```python
from build123d import *

# Parameters (mm, degrees)
SKETCH1_R           = 1
BOSS_EXTRUDE1_DEPTH = 1.5


with BuildPart() as part:
    # Sketch1 → Boss-Extrude1 (new, symmetric)
    with BuildSketch(Plane.XY):
        with BuildLine():
            Line((-0.022308457, 3.388443306), (-0.022308457, 3.09991973))
            ThreePointArc((-0.022308457, 3.09991973), (-0.270182803, 3.088203564), (-0.516325871, 3.056698807))
            Line((-0.516325871, 3.056698807), (-0.566427464, 3.340839061))
            ThreePointArc((-0.566427464, 3.340839061), (-0.583212597, 3.395348635), (-0.607768622, 3.446827136))
            ThreePointArc((-0.607768622, 3.446827136), (-0.806569619, 3.722605346), (-1.04548536, 3.964462178))
            ThreePointArc((-1.04548536, 3.964462178), (-1.402282588, 3.852739745), (-1.747418917, 3.708979257))
            ThreePointArc((-1.747418917, 3.708979257), (-1.774976418, 3.370134097), (-1.75, 3.031088913))
            ThreePointArc((-1.75, 3.031088913), (-1.735721264, 2.975869786), (-1.713541343, 2.923323754))
            Line((-1.713541343, 2.923323754), (-1.569279555, 2.673455008))
            ThreePointArc((-1.569279555, 2.673455008), (-1.778086953, 2.539371337), (-1.975500724, 2.389015883))
            Line((-1.975500724, 2.389015883), (-2.160960104, 2.610037765))
            ThreePointArc((-2.160960104, 2.610037765), (-2.202751242, 2.648851875), (-2.249756634, 2.681155551))
            ThreePointArc((-2.249756634, 2.681155551), (-2.559812453, 2.820585989), (-2.88764797, 2.910582279))
            ThreePointArc((-2.88764797, 2.910582279), (-3.140782217, 2.6354292), (-3.367798802, 2.3383608))
            ThreePointArc((-3.367798802, 2.3383608), (-3.222241717, 2.031133533), (-3.031088913, 1.75))
            ThreePointArc((-3.031088913, 1.75), (-2.991113602, 1.7093182), (-2.945632211, 1.674901963))
            Line((-2.945632211, 1.674901963), (-2.695763464, 1.530640175))
            ThreePointArc((-2.695763464, 1.530640175), (-2.80955414, 1.310116611), (-2.905341754, 1.081198083))
            Line((-2.905341754, 1.081198083), (-3.176465229, 1.179878957))
            ThreePointArc((-3.176465229, 1.179878957), (-3.232064471, 1.192597393), (-3.288924173, 1.197070502))
            ThreePointArc((-3.288924173, 1.197070502), (-3.627155608, 1.162792893), (-3.956067639, 1.076814208))
            ThreePointArc((-3.956067639, 1.076814208), (-4.037711787, 0.711957528), (-4.085779717, 0.341180455))
            ThreePointArc((-4.085779717, 0.341180455), (-3.806109951, 0.14789238), (-3.5, 0))
            ThreePointArc((-3.5, 0), (-3.445039465, -0.015243816), (-3.388443306, -0.022308457))
            Line((-3.388443306, -0.022308457), (-3.09991973, -0.022308457))
            ThreePointArc((-3.09991973, -0.022308457), (-3.088203564, -0.270182803), (-3.056698807, -0.516325871))
            Line((-3.056698807, -0.516325871), (-3.340839061, -0.566427464))
            ThreePointArc((-3.340839061, -0.566427464), (-3.395348635, -0.583212597), (-3.446827136, -0.607768622))
            ThreePointArc((-3.446827136, -0.607768622), (-3.722605346, -0.806569619), (-3.964462178, -1.04548536))
            ThreePointArc((-3.964462178, -1.04548536), (-3.852739745, -1.402282588), (-3.708979257, -1.747418917))
            ThreePointArc((-3.708979257, -1.747418917), (-3.370134097, -1.774976418), (-3.031088913, -1.75))
            ThreePointArc((-3.031088913, -1.75), (-2.975869786, -1.735721264), (-2.923323754, -1.713541343))
            Line((-2.923323754, -1.713541343), (-2.673455008, -1.569279555))
            ThreePointArc((-2.673455008, -1.569279555), (-2.539371337, -1.778086953), (-2.389015883, -1.975500724))
            Line((-2.389015883, -1.975500724), (-2.610037765, -2.160960104))
            ThreePointArc((-2.610037765, -2.160960104), (-2.648851875, -2.202751242), (-2.681155551, -2.249756634))
            ThreePointArc((-2.681155551, -2.249756634), (-2.820585989, -2.559812453), (-2.910582279, -2.88764797))
            ThreePointArc((-2.910582279, -2.88764797), (-2.6354292, -3.140782217), (-2.3383608, -3.367798802))
            ThreePointArc((-2.3383608, -3.367798802), (-2.031133533, -3.222241717), (-1.75, -3.031088913))
            ThreePointArc((-1.75, -3.031088913), (-1.7093182, -2.991113602), (-1.674901963, -2.945632211))
            Line((-1.674901963, -2.945632211), (-1.530640175, -2.695763464))
            ThreePointArc((-1.530640175, -2.695763464), (-1.310116611, -2.80955414), (-1.081198083, -2.905341754))
            Line((-1.081198083, -2.905341754), (-1.179878957, -3.176465229))
            ThreePointArc((-1.179878957, -3.176465229), (-1.192597393, -3.232064471), (-1.197070502, -3.288924173))
            ThreePointArc((-1.197070502, -3.288924173), (-1.162792893, -3.627155608), (-1.076814208, -3.956067639))
            ThreePointArc((-1.076814208, -3.956067639), (-0.711957528, -4.037711787), (-0.341180455, -4.085779717))
            ThreePointArc((-0.341180455, -4.085779717), (-0.14789238, -3.806109951), (0, -3.5))
            ThreePointArc((0, -3.5), (0.015243816, -3.445039465), (0.022308457, -3.388443306))
            Line((0.022308457, -3.388443306), (0.022308457, -3.09991973))
            ThreePointArc((0.022308457, -3.09991973), (0.270182803, -3.088203564), (0.516325871, -3.056698807))
            Line((0.516325871, -3.056698807), (0.566427464, -3.340839061))
            ThreePointArc((0.566427464, -3.340839061), (0.583212597, -3.395348635), (0.607768622, -3.446827136))
            ThreePointArc((0.607768622, -3.446827136), (0.806569619, -3.722605346), (1.04548536, -3.964462178))
            ThreePointArc((1.04548536, -3.964462178), (1.402282588, -3.852739745), (1.747418917, -3.708979257))
            ThreePointArc((1.747418917, -3.708979257), (1.774976418, -3.370134097), (1.75, -3.031088913))
            ThreePointArc((1.75, -3.031088913), (1.735721264, -2.975869786), (1.713541343, -2.923323754))
            Line((1.713541343, -2.923323754), (1.569279555, -2.673455008))
            ThreePointArc((1.569279555, -2.673455008), (1.778086953, -2.539371337), (1.975500724, -2.389015883))
            Line((1.975500724, -2.389015883), (2.160960104, -2.610037765))
            ThreePointArc((2.160960104, -2.610037765), (2.202751242, -2.648851875), (2.249756634, -2.681155551))
            ThreePointArc((2.249756634, -2.681155551), (2.559812453, -2.820585989), (2.88764797, -2.910582279))
            ThreePointArc((2.88764797, -2.910582279), (3.140782217, -2.6354292), (3.367798802, -2.3383608))
            ThreePointArc((3.367798802, -2.3383608), (3.222241717, -2.031133533), (3.031088913, -1.75))
            ThreePointArc((3.031088913, -1.75), (2.991113602, -1.7093182), (2.945632211, -1.674901963))
            Line((2.945632211, -1.674901963), (2.695763464, -1.530640175))
            ThreePointArc((2.695763464, -1.530640175), (2.80955414, -1.310116611), (2.905341754, -1.081198083))
            Line((2.905341754, -1.081198083), (3.176465229, -1.179878957))
            ThreePointArc((3.176465229, -1.179878957), (3.232064471, -1.192597393), (3.288924173, -1.197070502))
            ThreePointArc((3.288924173, -1.197070502), (3.627155608, -1.162792893), (3.956067639, -1.076814208))
            ThreePointArc((3.956067639, -1.076814208), (4.037711787, -0.711957528), (4.085779717, -0.341180455))
            ThreePointArc((4.085779717, -0.341180455), (3.806109951, -0.14789238), (3.5, 0))
            ThreePointArc((3.5, 0), (3.445039465, 0.015243816), (3.388443306, 0.022308457))
            Line((3.388443306, 0.022308457), (3.09991973, 0.022308457))
            ThreePointArc((3.09991973, 0.022308457), (3.088203564, 0.270182803), (3.056698807, 0.516325871))
            Line((3.056698807, 0.516325871), (3.340839061, 0.566427464))
            ThreePointArc((3.340839061, 0.566427464), (3.395348635, 0.583212597), (3.446827136, 0.607768622))
            ThreePointArc((3.446827136, 0.607768622), (3.722605346, 0.806569619), (3.964462178, 1.04548536))
            ThreePointArc((3.964462178, 1.04548536), (3.852739745, 1.402282588), (3.708979257, 1.747418917))
            ThreePointArc((3.708979257, 1.747418917), (3.370134097, 1.774976418), (3.031088913, 1.75))
            ThreePointArc((3.031088913, 1.75), (2.975869786, 1.735721264), (2.923323754, 1.713541343))
            Line((2.923323754, 1.713541343), (2.673455008, 1.569279555))
            ThreePointArc((2.673455008, 1.569279555), (2.539371337, 1.778086953), (2.389015883, 1.975500724))
            Line((2.389015883, 1.975500724), (2.610037765, 2.160960104))
            ThreePointArc((2.610037765, 2.160960104), (2.648851875, 2.202751242), (2.681155551, 2.249756634))
            ThreePointArc((2.681155551, 2.249756634), (2.820585989, 2.559812453), (2.910582279, 2.88764797))
            ThreePointArc((2.910582279, 2.88764797), (2.6354292, 3.140782217), (2.3383608, 3.367798802))
            ThreePointArc((2.3383608, 3.367798802), (2.031133533, 3.222241717), (1.75, 3.031088913))
            ThreePointArc((1.75, 3.031088913), (1.7093182, 2.991113602), (1.674901963, 2.945632211))
            Line((1.674901963, 2.945632211), (1.530640175, 2.695763464))
            ThreePointArc((1.530640175, 2.695763464), (1.310116611, 2.80955414), (1.081198083, 2.905341754))
            Line((1.081198083, 2.905341754), (1.179878957, 3.176465229))
            ThreePointArc((1.179878957, 3.176465229), (1.192597393, 3.232064471), (1.197070502, 3.288924173))
            ThreePointArc((1.197070502, 3.288924173), (1.162792893, 3.627155608), (1.076814208, 3.956067639))
            ThreePointArc((1.076814208, 3.956067639), (0.711957528, 4.037711787), (0.341180455, 4.085779717))
            ThreePointArc((0.341180455, 4.085779717), (0.14789238, 3.806109951), (0, 3.5))
            ThreePointArc((0, 3.5), (-0.015243816, 3.445039465), (-0.022308457, 3.388443306))
        make_face()
        Circle(SKETCH1_R, mode=Mode.SUBTRACT)
    extrude(amount=BOSS_EXTRUDE1_DEPTH, both=True)


solid = part.part
```
Read the model definition and answer for the solid it produces. Units are mm, in the model's axes. Round coordinates to 2 decimals unless told otherwise and drop trailing zeros. Write each loop counter-clockwise with the first axis right and the second up, starting at its lowest first coordinate (ties: lowest second). Pieces come first, ordered by that corner, then holes. Notation, with made-up numbers: (28, 49.5) - (50, 49.5) arc R16 cw to (50, 56.5) - close; hole circle Ø9 at (67, -7). An arc over 180 degrees is marked (long way). One line per item, written item: value.
Q1. For a pull along Y with two mould halves and no side action, classify faces 1 (the flat face through (1, -1, -1.5)), 2 (the cylindrical face through (0, -1, 0)) as pulls with the +Y half, pulls with the -Y half, needs draft (parallel to the pull), parting line crosses it, or undercut.
The answers:
face 1: needs draft
face 2: undercut
Q2. Straight lines are drawn through the part: line 1 (Y direction, x = -3.25, z = 0.2); line 2 (Y direction, x = -3, z = -0.9); line 3 (X direction, y = -0.25, z = 0.55). For each, find the intervals that lie inside material, in ascending order. Write a range as from..to.
The answers:
line 1: y = -1.77..-0.55, -0.02..1.19, 2.08..2.5
line 2: y = -1.74..1.12, 1.72..2.79
line 3: x = -3.09..-0.97, 0.97..3.97
Q3. Find section A-A (x = 0.75). Determine the outline of the cut face in (y, z).
The answers:
outline: (-3.65, -1.5) - (-0.66, -1.5) - (-0.66, 1.5) - (-3.65, 1.5) - close; (0.66, -1.5) - (4.03, -1.5) - (4.03, 1.5) - (0.66, 1.5) - close
